The listing builds one solid part. Answer for the finished solid, in the listing's coordinates (mm). Give positions to 0.01 mm unless a question says otherwise; leave off trailing zeros. Loops run counter-clockwise (first coordinate to the right, second up) from the corner with the lowest first, then second, coordinate; pieces in that order, holes last. Notation, with made-up numbers: (64.25, 65) - (69.25, 65) arc R11 ccw to (69.25, 72) - close; hole circle Ø8 at (49, -27.5). An arc over 180 degrees is marked (long way). Write item = value, one per line. Start each with the question number.
1) The part is cut by section A-A on y = 0. Write down the section's boundary in (x, z).
2) Flat-ended cylindrical pins translate along their axes: P1, Ø6.5, axis at x = -52.5, y = 0, coming from the -Z side; P2, Ø4, axis at x = 45, z = 5, coming from the +Y side; P3, Ø2, axis at x = 33.5, z = 4.5, coming from the -Y side; P4, Ø1, axis at y = 43, z = 4.5, coming from the +X side. Find the tip coordinate at first contact, or state that the pin passes through.
3) The part is cut by section D-D on z = 5.5. State how many separate pieces and enclosed holes the cut face has, plus the area to 3 significant figures.
4) The part is cut by section C-C on x = -25.5. Write down the section's boundary in (y, z), plus the area to 3 significant figures.
5) Consider probe 1 along Y at (x, z) = (0, 4.25); probe 2 along Y at (x, z) = (35.5, 3.5); probe 3 along Y at (x, z) = (38, 5). Determine where each line is inside the solid, lowest interval first.
6) The mould has two halves that part along X. Classify faces 1 (the cylindrical face through (-59.94, 2.64, 3.45)), 2 (the flat face through (12, -26, 7)), 3 (the cylindrical face through (-0.521, 38.966, 3.549)): +X half, -X half, draft (parallel to the pull), parting line (faces both ways), or undercut.
from build123d import *

# Parameters (mm, degrees)
CROQUIS1_R              = 60
SALIENTE_EXTRUIR1_DEPTH = 7
CROQUIS2_R              = 27
CORTAR_EXTRUIR1_DEPTH   = 8
CROQUIS3_R              = 4
CORTAR_EXTRUIR2_DEPTH   = 8
CROQUIS5_R              = 2.5
CORTAR_EXTRUIR3_DEPTH   = 8


with BuildPart() as part:
    # Croquis1 → Saliente-Extruir1 (new body)
    with BuildSketch(Plane.XY):
        Circle(CROQUIS1_R)
    extrude(amount=SALIENTE_EXTRUIR1_DEPTH)

    # Croquis2 → Cortar-Extruir1 (cut, through all)
    with BuildSketch(Plane.XY.offset(7)):
        Circle(CROQUIS2_R)
    extrude(amount=-CORTAR_EXTRUIR1_DEPTH, mode=Mode.SUBTRACT)

    # Croquis3 → Cortar-Extruir2 (cut, through all)
    with BuildSketch(Plane.XY.offset(7)):
        with Locations((0, 35)):
            Circle(CROQUIS3_R)
        with Locations((35, 0)):
            Circle(CROQUIS3_R)
        with Locations((0, -35)):
            Circle(CROQUIS3_R)
        with Locations((-35, 0)):
            Circle(CROQUIS3_R)
    extrude(amount=-CORTAR_EXTRUIR2_DEPTH, mode=Mode.SUBTRACT)

    # Croquis5 → Cortar-Extruir3 (cut, through all)
    with BuildSketch(Plane.XY.offset(7)):
        with Locations((37.123106012, 37.123106012)):
            Circle(CROQUIS5_R)
        with Locations((52.5, 0)):
            Circle(CROQUIS5_R)
        with Locations((37.123106012, -37.123106012)):
            Circle(CROQUIS5_R)
        with Locations((-52.5, 0)):
            Circle(CROQUIS5_R)
        with Locations((-37.123106012, 37.123106012)):
            Circle(CROQUIS5_R)
        with Locations((0, 52.5)):
            Circle(CROQUIS5_R)
        with Locations((0, -52.5)):
            Circle(CROQUIS5_R)
        with Locations((-37.123106012, -37.123106012)):
            Circle(CROQUIS5_R)
    extrude(amount=-CORTAR_EXTRUIR3_DEPTH, mode=Mode.SUBTRACT)


solid = part.part
Answer below:
q1.outline = (-60, 0) - (-55, 0) - (-55, 7) - (-60, 7) - close; (-50, 0) - (-39, 0) - (-39, 7) - (-50, 7) - close; (-31, 0) - (-27, 0) - (-27, 7) - (-31, 7) - close; (27, 0) - (31, 0) - (31, 7) - (27, 7) - close; (39, 0) - (50, 0) - (50, 7) - (39, 7) - close; (55, 0) - (60, 0) - (60, 7) - (55, 7) - close
q2.P1 = 0
q2.P2 = 41.84
q2.P3 = -50.44
q2.P4 = 42.35
q3.separate_pieces = 1
q3.enclosed_holes = 13
q3.area = 8,660 mm2
q4.outline = (-54.31, 0) - (-8.87, 0) - (-8.87, 7) - (-54.31, 7) - close; (8.87, 0) - (54.31, 0) - (54.31, 7) - (8.87, 7) - close
q4.area = 636 mm2
q5.probe_1 = -60 to -55, -50 to -39, -31 to -27, 27 to 31, 39 to 50, 55 to 60
q5.probe_2 = -48.37 to -39.02, -35.22 to -3.97, 3.97 to 35.22, 39.02 to 48.37
q5.probe_3 = -46.43 to -39.46, -34.78 to -2.65, 2.65 to 34.78, 39.46 to 46.43
q6.face_1 = parting line
q6.face_2 = draft
q6.face_3 = undercut
